The model under review builds one solid part; all positions refer to its coordinate system, in mm. A direction names the side the tool comes from. Coordinates: 2 decimals unless noted, no trailing zeros. Write each loop counter-clockwise with the first axis right and the second up, starting at its lowest first coordinate (ties: lowest second). Pieces come first, ordered by that corner, then holes. Notation, with made-up numbers: M 12.25,34.5 L 38.25,34.5 A18 ccw 38.25,44.5 Z; hole C 36,63 d3. An arc over 180 degrees is marked long. Answer as CSV lines item,"result". Start each with the question number.
from build123d import *

# Parameters (mm, degrees)
F0_R     = 2.5
F1_DEPTH = 20
F2_DEPTH = 12
F3_R     = 5


with BuildPart() as f1:
    # F0 (on Top) → F1 (new body)
    with BuildSketch(Plane.XY):
        with BuildLine():
            ThreePointArc((6.8334705864, -3.0909027395), (5.8642916103, 0.2220330494), (6.5801871048, 3.5987689097))
            ThreePointArc((6.5801871048, 3.5987689097), (5.0988546193, 5.500152868), (3.0909027395, 6.8334705864))
            ThreePointArc((3.0909027395, 6.8334705864), (-0.2220330494, 5.8642916103), (-3.5987689097, 6.5801871048))
            ThreePointArc((-3.5987689097, 6.5801871048), (-5.500152868, 5.0988546193), (-6.8334705864, 3.0909027395))
            ThreePointArc((-6.8334705864, 3.0909027395), (-6.1071411443, 1.3658616264), (-5.8592325951, -0.489364142))
            ThreePointArc((-5.8592325951, -0.489364142), (-6.0418306344, -2.0853100539), (-6.5801871048, -3.5987689097))
            ThreePointArc((-6.5801871048, -3.5987689097), (-5.0988546193, -5.500152868), (-3.0909027395, -6.8334705864))
            ThreePointArc((-3.0909027395, -6.8334705864), (0.2220330494, -5.8642916103), (3.5987689097, -6.5801871048))
            ThreePointArc((3.5987689097, -6.5801871048), (5.500152868, -5.0988546193), (6.8334705864, -3.0909027395))
        make_face()
        Circle(F0_R, mode=Mode.SUBTRACT)
        with BuildLine():
            ThreePointArc((-3.5987689097, 6.5801871048), (-0.2220330494, 5.8642916103), (3.0909027395, 6.8334705864))
            ThreePointArc((3.0909027395, 6.8334705864), (-0.283760713, 7.4946300681), (-3.5987689097, 6.5801871048))
        make_face()
        with BuildLine():
            ThreePointArc((6.8334705864, -3.0909027395), (7.3314742514, -1.5809760596), (7.5, 0))
            ThreePointArc((7.5, 0), (7.2664091299, 1.8572286765), (6.5801871048, 3.5987689097))
            ThreePointArc((6.5801871048, 3.5987689097), (5.8642916103, 0.2220330494), (6.8334705864, -3.0909027395))
        make_face()
        with BuildLine():
            ThreePointArc((-3.0909027395, -6.8334705864), (0.283760713, -7.4946300681), (3.5987689097, -6.5801871048))
            ThreePointArc((3.5987689097, -6.5801871048), (0.2220330494, -5.8642916103), (-3.0909027395, -6.8334705864))
        make_face()
        with BuildLine():
            ThreePointArc((-5.8592325951, -0.489364142), (-6.1071411443, 1.3658616264), (-6.8334705864, 3.0909027395))
            ThreePointArc((-6.8334705864, 3.0909027395), (-7.4946300681, -0.283760713), (-6.5801871048, -3.5987689097))
            ThreePointArc((-6.5801871048, -3.5987689097), (-6.0418306344, -2.0853100539), (-5.8592325951, -0.489364142))
        make_face()
    extrude(amount=F1_DEPTH)

    # F0 (on Top) → F2 (join)
    with BuildSketch(Plane.XY):
        with BuildLine():
            ThreePointArc((-6.5229662777, -13.7922181567), (-5.8475768655, -9.7995981798), (-3.0909027395, -6.8334705864))
            ThreePointArc((-3.0909027395, -6.8334705864), (-5.0988546193, -5.500152868), (-6.5801871048, -3.5987689097))
            ThreePointArc((-6.5801871048, -3.5987689097), (-9.3293758522, -6.5718355247), (-13.2594952145, -7.5471947736))
            ThreePointArc((-13.2594952145, -7.5471947736), (-8.751081206, -9.4398231008), (-6.5229662777, -13.7922181567))
        make_face()
        with BuildLine():
            ThreePointArc((6.5801871048, 3.5987689097), (7.2664091299, 1.8572286765), (7.5, 0))
            ThreePointArc((7.5, 0), (7.3314742514, -1.5809760596), (6.8334705864, -3.0909027395))
            ThreePointArc((6.8334705864, -3.0909027395), (9.7995980718, -5.8475768122), (13.7922179176, -6.5229663073))
            ThreePointArc((13.7922179176, -6.5229663073), (18.2189691424, -4.1902310429), (19.9907391968, 0.489364142))
            ThreePointArc((19.9907391968, 0.489364142), (19.9894743232, 0.6230539717), (19.985680155, 0.7566959365))
            ThreePointArc((19.985680155, 0.7566959365), (17.9449438052, 5.4617772682), (13.2594951602, 7.5471947762))
            ThreePointArc((13.2594951602, 7.5471947762), (9.3293758288, 6.5718355109), (6.5801871048, 3.5987689097))
        make_face()
        with BuildLine():
            ThreePointArc((13.7922179176, -6.5229663073), (9.7995980718, -5.8475768122), (6.8334705864, -3.0909027395))
            ThreePointArc((6.8334705864, -3.0909027395), (5.500152868, -5.0988546193), (3.5987689097, -6.5801871048))
            ThreePointArc((3.5987689097, -6.5801871048), (6.4849940801, -9.1863643112), (7.5551174429, -12.9249858959))
            ThreePointArc((7.5551174429, -12.9249858959), (7.5531364952, -13.0922875721), (7.547194763, -13.2594954392))
            ThreePointArc((7.547194763, -13.2594954392), (9.4398229424, -8.7510813768), (13.7922179176, -6.5229663073))
        make_face()
        with BuildLine():
            ThreePointArc((6.8334705864, -3.0909027395), (5.8642916103, 0.2220330494), (6.5801871048, 3.5987689097))
            ThreePointArc((6.5801871048, 3.5987689097), (5.0988546193, 5.500152868), (3.0909027395, 6.8334705864))
            ThreePointArc((3.0909027395, 6.8334705864), (-0.2220330494, 5.8642916103), (-3.5987689097, 6.5801871048))
            ThreePointArc((-3.5987689097, 6.5801871048), (-5.500152868, 5.0988546193), (-6.8334705864, 3.0909027395))
            ThreePointArc((-6.8334705864, 3.0909027395), (-6.1071411443, 1.3658616264), (-5.8592325951, -0.489364142))
            ThreePointArc((-5.8592325951, -0.489364142), (-6.0418306344, -2.0853100539), (-6.5801871048, -3.5987689097))
            ThreePointArc((-6.5801871048, -3.5987689097), (-5.0988546193, -5.500152868), (-3.0909027395, -6.8334705864))
            ThreePointArc((-3.0909027395, -6.8334705864), (0.2220330494, -5.8642916103), (3.5987689097, -6.5801871048))
            ThreePointArc((3.5987689097, -6.5801871048), (5.500152868, -5.0988546193), (6.8334705864, -3.0909027395))
        make_face()
        Circle(F0_R, mode=Mode.SUBTRACT)
        with BuildLine():
            ThreePointArc((6.8334705864, -3.0909027395), (7.3314742514, -1.5809760596), (7.5, 0))
            ThreePointArc((7.5, 0), (7.2664091299, 1.8572286765), (6.5801871048, 3.5987689097))
            ThreePointArc((6.5801871048, 3.5987689097), (5.8642916103, 0.2220330494), (6.8334705864, -3.0909027395))
        make_face()
        with BuildLine():
            ThreePointArc((7.5551174429, -12.9249858959), (6.4849940801, -9.1863643112), (3.5987689097, -6.5801871048))
            ThreePointArc((3.5987689097, -6.5801871048), (0.283760713, -7.4946300681), (-3.0909027395, -6.8334705864))
            ThreePointArc((-3.0909027395, -6.8334705864), (-5.8475768655, -9.7995981798), (-6.5229662777, -13.7922181567))
            ThreePointArc((-6.5229662777, -13.7922181567), (-4.0892275286, -18.3065626187), (0.7566938759, -19.9856802331))
            ThreePointArc((0.7566938759, -19.9856802331), (5.4617764365, -17.9449446291), (7.547194763, -13.2594954392))
            ThreePointArc((7.547194763, -13.2594954392), (7.5531364952, -13.0922875721), (7.5551174429, -12.9249858959))
        make_face()
        with BuildLine():
            ThreePointArc((3.0909027395, 6.8334705864), (5.0988546193, 5.500152868), (6.5801871048, 3.5987689097))
            ThreePointArc((6.5801871048, 3.5987689097), (9.3293758288, 6.5718355109), (13.2594951602, 7.5471947762))
            ThreePointArc((13.2594951602, 7.5471947762), (8.7510812527, 9.4398230574), (6.5229663, 13.7922179762))
            ThreePointArc((6.5229663, 13.7922179762), (6.5630207977, 13.3594238901), (6.5763891589, 12.9249858959))
            ThreePointArc((6.5763891589, 12.9249858959), (5.6434228364, 9.4158843604), (3.0909027395, 6.8334705864))
        make_face()
        with BuildLine():
            ThreePointArc((-3.5987689097, 6.5801871048), (-0.283760713, 7.4946300681), (3.0909027395, 6.8334705864))
            ThreePointArc((3.0909027395, 6.8334705864), (5.6434228364, 9.4158843604), (6.5763891589, 12.9249858959))
            ThreePointArc((6.5763891589, 12.9249858959), (6.5630207977, 13.3594238901), (6.5229663, 13.7922179762))
            ThreePointArc((6.5229663, 13.7922179762), (4.0892269422, 18.3065631176), (-0.7566955961, 19.9856801679))
            ThreePointArc((-0.7566955961, 19.9856801679), (-5.4617770309, 17.9449440403), (-7.5471947607, 13.2594954872))
            ThreePointArc((-7.5471947607, 13.2594954872), (-6.5718355942, 9.3293759697), (-3.5987689097, 6.5801871048))
        make_face()
        with BuildLine():
            ThreePointArc((-6.8334705864, 3.0909027395), (-5.500152868, 5.0988546193), (-3.5987689097, 6.5801871048))
            ThreePointArc((-3.5987689097, 6.5801871048), (-6.5718355942, 9.3293759697), (-7.5471947607, 13.2594954872))
            ThreePointArc((-7.5471947607, 13.2594954872), (-9.4398229383, 8.7510813813), (-13.7922179532, 6.5229663029))
            ThreePointArc((-13.7922179532, 6.5229663029), (-9.7995980879, 5.8475768202), (-6.8334705864, 3.0909027395))
        make_face()
        with BuildLine():
            ThreePointArc((-6.5801871048, -3.5987689097), (-7.4946300681, -0.283760713), (-6.8334705864, 3.0909027395))
            ThreePointArc((-6.8334705864, 3.0909027395), (-9.7995980879, 5.8475768202), (-13.7922179532, 6.5229663029))
            ThreePointArc((-13.7922179532, 6.5229663029), (-18.3065631087, 4.0892269526), (-19.9856801681, -0.756695592))
            ThreePointArc((-19.9856801681, -0.756695592), (-17.9449439456, -5.4617771265), (-13.2594952145, -7.5471947736))
            ThreePointArc((-13.2594952145, -7.5471947736), (-9.3293758522, -6.5718355247), (-6.5801871048, -3.5987689097))
        make_face()
        with BuildLine():
            ThreePointArc((-5.8592325951, -0.489364142), (-6.1071411443, 1.3658616264), (-6.8334705864, 3.0909027395))
            ThreePointArc((-6.8334705864, 3.0909027395), (-7.4946300681, -0.283760713), (-6.5801871048, -3.5987689097))
            ThreePointArc((-6.5801871048, -3.5987689097), (-6.0418306344, -2.0853100539), (-5.8592325951, -0.489364142))
        make_face()
        with BuildLine():
            ThreePointArc((-3.0909027395, -6.8334705864), (0.283760713, -7.4946300681), (3.5987689097, -6.5801871048))
            ThreePointArc((3.5987689097, -6.5801871048), (0.2220330494, -5.8642916103), (-3.0909027395, -6.8334705864))
        make_face()
        with BuildLine():
            ThreePointArc((-3.5987689097, 6.5801871048), (-0.2220330494, 5.8642916103), (3.0909027395, 6.8334705864))
            ThreePointArc((3.0909027395, 6.8334705864), (-0.283760713, 7.4946300681), (-3.5987689097, 6.5801871048))
        make_face()
    extrude(amount=F2_DEPTH)

    # F3
    f3_edges = [f1.edges().sort_by_distance(p)[0] for p in [
        (-19.98568, -0.756695, 12),
        (-19.98568, -0.756695, 0),
    ]]
    fillet(f3_edges, radius=F3_R)


solid = f1.part
1) To check wall thickness, follow line 1 (Y direction, x = 0, z = 5.5); line 2 (Y direction, x = 0, z = 14.5); line 3 (Z direction, x = -2, y = -10.5). State the ranges of each line that lie inside material, in increasing order. Write a range as [from, to].
2) Tool access review of faces 4 (the flat face through (0, 8, 12)), 5 (the flat face through (-2, -2, 0)): name each direction out of +Z, -Z, +X, -X, +Y, -Y from which nothing blocks a thin tool from reaching the whole face with its end or side.
3) Mouldability with a two-part tool opening along Y and no side actions: class faces 1 (the cylindrical face through (9.393, -8.803, 5.986)), 2 (the cylindrical face through (-0.54, -2.44, 9.86)), 3 (the flat face through (-2, 2, 20)) as +Y half, -Y half, draft (parallel to the pull), parting line (faces both ways), or undercut.
4) Take a section at A-A on z = 16.5. Give the boundary of the cut face in (x, y).
5) Clearance check with flat-ended pins moving along their axes: pin 1 Ø6 at (y, z) = (-3, 4) entering from +X; pin 2 Ø3 at (x, y) = (0, 0) entering from -Z; pin 3 Ø8 at (y, z) = (-14.5, 6.5) entering from +X; pin 4 Ø10 at (y, z) = (15, 15) entering from +X. State where each tip first meets the part, or that it passes through.
Results:
1,line 1,"y = [-19.97, -2.5], [2.5, 19.97]"
1,line 2,"y = [-7.5, -2.5], [2.5, 7.5]"
1,line 3,"z = [0, 12]"
2,face 4,"+Z"
2,face 5,"-Z, +X, -X, +Y, -Y"
3,face 1,"-Y half"
3,face 2,"undercut"
3,face 3,"draft"
4,outline,"C 0,0 d15; hole C 0,0 d5"
5,pin 1,"stops at x = 19.96"
5,pin 2,"passes through"
5,pin 3,"stops at x = 8.25"
5,pin 4,"stops at x = 5.4"
